Job drawing, mm, ordinate dimensions from the low corner. One solid piece. Round coordinates to 2 decimals unless told otherwise and drop trailing zeros. Order: outer loops, then holes, each group sorted by start corner. A loop starts at its lowest first (then second) coordinate and runs counter-clockwise, first axis right, second up. Notation, with made-up numbers: (15, 65.5) -> (38, 65.5) arc R10 cw to (38, 78.5) -> close; hole circle Ø9 at (23, -37.75). An arc over 180 degrees is marked (long way). Return JSON: item names as keys, results as strings. Group by question number.
Q1. Cut at D-D (x = 169.5). Write the cut outline in (y, z), then the cut area to 4 significant figures.
Q2. Probe line 1 along X through (y, z) = (4.25, 81.5); line 2 along X through (y, z) = (8.5, 24); line 3 along Z through (x, y) = (153, 14.75). List the from-to ranges inside material, lowest first.
Q3. Cut at B-B (y = 7). Write the cut outline in (x, z), then the cut area to 3 significant figures.
Q4. Cut at A-A (z = 267.5). Write the cut outline in (x, y).
Q5. Flat gauge pins, fed straight in: pin 1 (2 mm diameter, centred on y = 8.5, z = 239, fed in from -X); pin 2 (8 mm diameter, centred on y = 6.5, z = 158, fed in from -X); pin 3 (6 mm diameter, centred on x = 165.5, y = 14, fed in from +Z). Where does each tip first touch, or does it go through?
Q6. Cut at C-C (z = 44.5). Write the cut outline in (x, y), then the cut area to 3 significant figures.
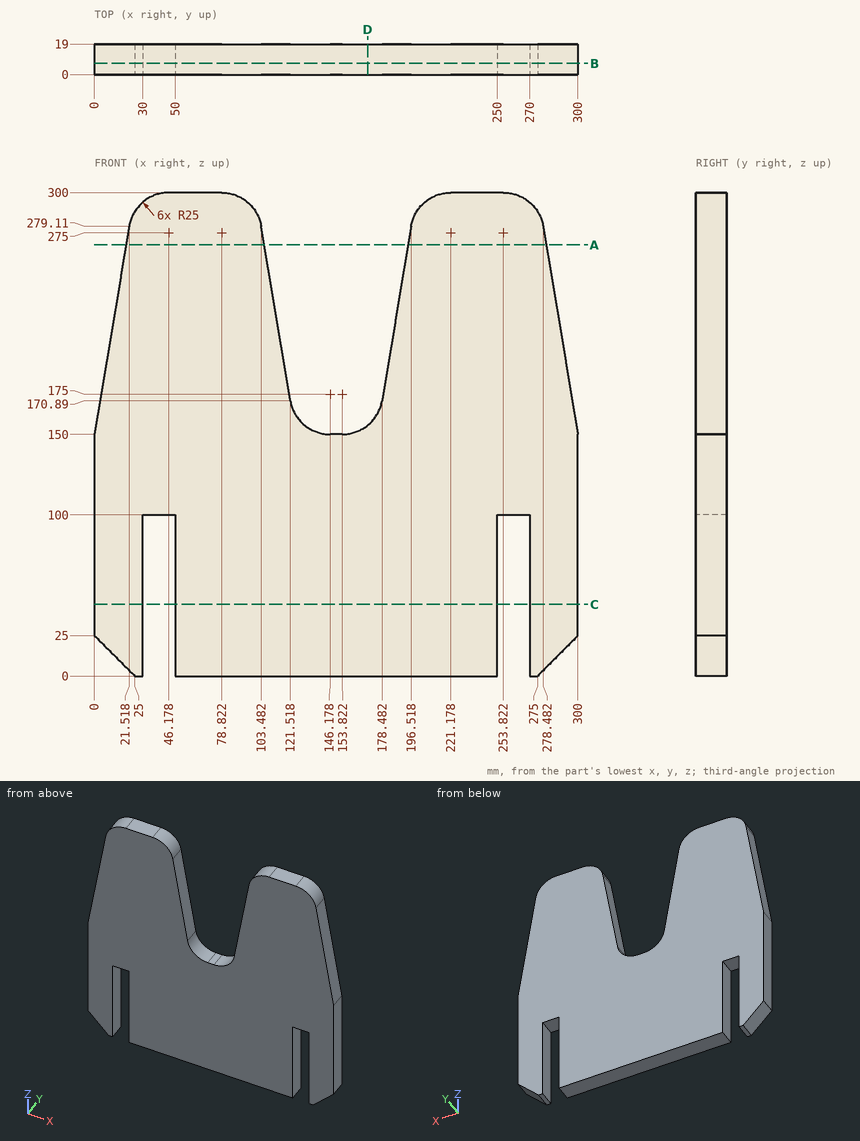
Solution:
{
 "1": {"outline": "(0, 0) -> (19, 0) -> (19, 155.53) -> (0, 155.53) -> close", "area": "2,955 mm²"},
 "2": {"line 1": "x = 0 to 30, 50 to 250, 270 to 300", "line 2": "x = 1 to 30, 50 to 250, 270 to 299", "line 3": "z = 0 to 150"},
 "3": {"outline": "(0, 25) -> (25, 0) -> (30, 0) -> (30, 100) -> (50, 100) -> (50, 0) -> (250, 0) -> (250, 100) -> (270, 100) -> (270, 0) -> (275, 0) -> (300, 25) -> (300, 150) -> (278.48, 279.11) arc R25 ccw to (253.82, 300) -> (221.18, 300) arc R25 ccw to (196.52, 279.11) -> (178.48, 170.89) arc R25 cw to (153.82, 150) -> (146.18, 150) arc R25 cw to (121.52, 170.89) -> (103.48, 279.11) arc R25 ccw to (78.82, 300) -> (46.18, 300) arc R25 ccw to (21.52, 279.11) -> (0, 150) -> close", "area": "70,200 mm²"},
 "4": {"outline": "(19.58, 0) -> (105.42, 0) -> (105.42, 19) -> (19.58, 19) -> close; (194.58, 0) -> (280.42, 0) -> (280.42, 19) -> (194.58, 19) -> close"},
 "5": {"pin 1": "stops at x = 14.67", "pin 2": "stops at x = 0.67", "pin 3": "stops at z = 154.76"},
 "6": {"outline": "(0, 0) -> (30, 0) -> (30, 19) -> (0, 19) -> close; (50, 0) -> (250, 0) -> (250, 19) -> (50, 19) -> close; (270, 0) -> (300, 0) -> (300, 19) -> (270, 19) -> close", "area": "4,940 mm²"}
}
